from build123d import *

# Parameters (mm, degrees)
BOSS_EXTRUDE1_DEPTH = 5.08
SKETCH2_R           = 2.54
BOSS_EXTRUDE2_DEPTH = 19.05


with BuildPart() as part:
    # Sketch1 → Boss-Extrude1 (new body)
    with BuildSketch(Plane.XY):
        with BuildLine():
            Line((3.465176556, 17.167746033), (63.408488693, 5.068652798))
            ThreePointArc((63.408488693, 5.068652798), (67.556291682, 0), (63.408488693, -5.068652798))
            Line((63.408488693, -5.068652798), (3.465176556, -17.167746033))
            ThreePointArc((3.465176556, -17.167746033), (-17.513964497, 0), (3.465176556, 17.167746033))
        make_face()
        Polygon((12.70363461, 0), (6.351817305, 11.001670293), (-6.351817305, 11.001670293), (-12.70363461, 0), (-6.351817305, -11.001670293), (6.351817305, -11.001670293), align=None, mode=Mode.SUBTRACT)
    extrude(amount=BOSS_EXTRUDE1_DEPTH)

    # Sketch2 → Boss-Extrude2 (add)
    with BuildSketch(Plane.XY.offset(5.08)):
        with Locations(Location((62.385420387, 0, 0), (0, 0, 180))):
            Circle(SKETCH2_R)
    extrude(amount=BOSS_EXTRUDE2_DEPTH)


solid = part.part
For this review, take the finished solid that the model builds, in its own axes (mm). A direction names the side the tool comes from. Coordinates: 2 decimals unless noted, no trailing zeros. Order: outer loops, then holes, each group sorted by start corner. A loop starts at its lowest first (then second) coordinate and runs counter-clockwise, first axis right, second up. Notation, with made-up numbers: (37.5, 89) - (56.5, 89) arc R14 ccw to (56.5, 111) - close; hole circle Ø9 at (76, -28.5). An arc over 180 degrees is marked (long way). Answer as CSV lines item,"result". Start each with the question number.
1) Draft analysis for pull direction Y (two halves, no side actions). For faces 1 (the flat face through (9.572, 5.424, 2.504)), 2 (the flat face through (26, 0, 5.08)), 3 (the cylindrical face through (67.555, 0.099, 2.504)), state which applies: +Y half, -Y half, draft (parallel to the pull), parting line (faces both ways), or undercut.
2) Add section B-B (y = -10). State the section outline as (x, z) points, then the cut area to 3 significant figures.
3) Insertion check: P1, Ø17.5, axis at x = 32, y = -3, coming from the +Z side; P2, Ø1.5, axis at x = -1, z = 2.5, coming from the -Y side; P3, Ø1.5, axis at x = 1.5, z = 4, coming from the +Y side. Each pin has a flat end and moves straight along its axis. Give the tip position at first contact, or say it passes through.
4) To check wall thickness, follow line 1 along Z through (x, y) = (38.5, -6); line 2 along Y through (x, z) = (57, 3); line 3 along Y through (x, z) = (63.5, 2). State the ranges of each line that lie inside material, in increasing order. Write a range as [from, to].
5) Add section D-D (y = -1). State the section outline as (x, z) points.
6) Add section C-C (z = 22.25). State the section outline as (x, y) points, then the cut area to 3 significant figures.
7) Add section A-A (x = 0). State the section outline as (y, z) points, then the cut area to 3 significant figures.
8) Machinability: for faces 4 (the flat face through (-9.572, -5.424, 2.504)), 5 (the flat face through (33.017, 11.203, 2.504)), 6 (the cylindrical face through (59.96, -0.76, 14.47)), which of the approach directions +Z, -Z, +X, -X, +Y, -Y give a long, thin tool a straight path to every point of the face, cutting with its end or side? Answer none if there is none.
Result:
1,face 1,"undercut"
1,face 2,"draft"
1,face 3,"parting line"
2,outline,"(-14.38, 0) - (-6.93, 0) - (-6.93, 5.08) - (-14.38, 5.08) - close; (6.93, 0) - (38.98, 0) - (38.98, 5.08) - (6.93, 5.08) - close"
2,area,"201 mm^2"
3,P1,"z = 5.08"
3,P2,"y = -17.51"
3,P3,"y = 17.5"
4,line 1,"[0, 5.08]"
4,line 2,"[-6.36, 6.36]"
4,line 3,"[-5.05, 5.05]"
5,outline,"(-17.49, 0) - (-12.13, 0) - (-12.13, 5.08) - (-17.49, 5.08) - close; (12.13, 0) - (67.46, 0) - (67.46, 5.08) - (64.72, 5.08) - (64.72, 24.13) - (60.05, 24.13) - (60.05, 5.08) - (12.13, 5.08) - close"
6,outline,"circle Ø5.08 at (62.39, 0)"
6,area,"20.3 mm^2"
7,outline,"(-17.51, 0) - (-11, 0) - (-11, 5.08) - (-17.51, 5.08) - close; (11, 0) - (17.51, 0) - (17.51, 5.08) - (11, 5.08) - close"
7,area,"66.2 mm^2"
8,face 4,"+Z, -Z"
8,face 5,"+Z, -Z, +X, +Y"
8,face 6,"+Z"
